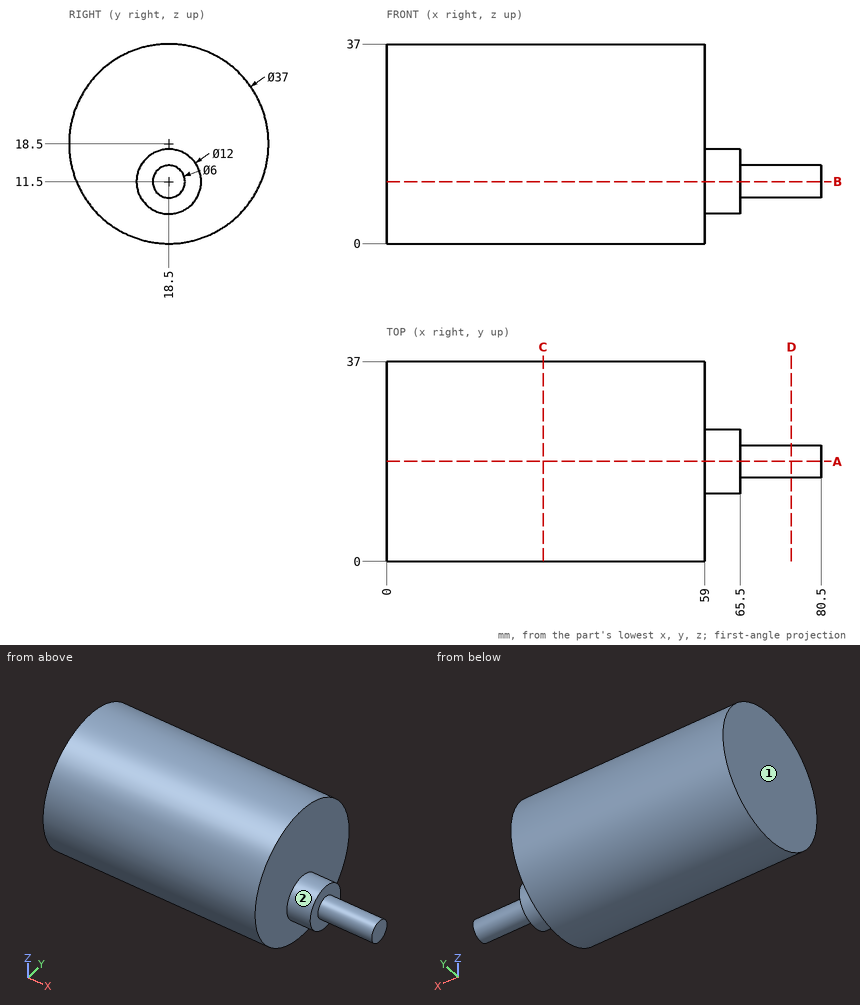
The drawing under review shows one solid part. Ordinate dimensions are in mm from its lowest x, y, z. A direction names the side the tool comes from. Coordinates: 2 decimals unless noted, no trailing zeros. Write each loop counter-clockwise with the first axis right and the second up, starting at its lowest first coordinate (ties: lowest second). Pieces come first, ordered by that corner, then holes. Notation, with made-up numbers: M 67.25,45 L 85.25,45 A18 cw 85.25,64 Z; hole C -33,-1 d1. An arc over 180 degrees is marked long. Put each result on its own line as item: value.
1) Add section A-A on y = 18.5. Give the boundary of the cut face in (x, z), then the cut area to 3 significant figures.
Computed:
outline: M 0,0 L 59,0 L 59,5.5 L 65.5,5.5 L 65.5,8.5 L 80.5,8.5 L 80.5,14.5 L 65.5,14.5 L 65.5,17.5 L 59,17.5 L 59,37 L 0,37 Z
area: 2,350 mm2
2) Add section C-C on x = 29. Give the boundary of the cut face in (y, z), then the cut area to 3 significant figures.
Computed:
outline: C 18.5,18.5 d37
area: 1,080 mm2
3) Add section D-D on x = 75. Give the boundary of the cut face in (y, z).
Computed:
outline: C 18.5,11.5 d6
4) Add section B-B on z = 11.5. Give the boundary of the cut face in (x, y).
Computed:
outline: M 0,1.38 L 59,1.38 L 59,12.5 L 65.5,12.5 L 65.5,15.5 L 80.5,15.5 L 80.5,21.5 L 65.5,21.5 L 65.5,24.5 L 59,24.5 L 59,35.62 L 0,35.62 Z
5) Clearance check with flat-ended pins moving along their axes: pin 1 Ø11 at (y, z) = (25.5, 25.5) entering from +X; pin 2 Ø3 at (x, z) = (23, 21.5) entering from +Y; pin 3 Ø6 at (x, z) = (9.5, 10) entering from -Y; pin 4 Ø9.5 at (y, z) = (16, 9.5) entering from +X. State where each tip first meets the part, or that it passes through.
Computed:
pin 1: stops at x = 59
pin 2: stops at y = 36.94
pin 3: stops at y = 0.84
pin 4: stops at x = 80.5
6) Wall thickness on probe 1 along X at (y, z) = (7, 30); probe 2 along X at (y, z) = (23, 14.5); probe 3 along Y at (x, z) = (15.5, 25.5): over which ranges is each line inside the solid? List them lowest first. Write a range as [from, to].
Computed:
probe 1: x = [0, 59]
probe 2: x = [0, 65.5]
probe 3: y = [1.38, 35.62]
7) For the marked faces 1 and 2, list the 3-axis set-ups (+Z, -Z, +X, -X, +Y, -Y) from which the entire face can be reached by the end or side of a thin tool; tool diameter is ignored.
Computed:
face 1: +Z, -Z, -X, +Y, -Y
face 2: +X
